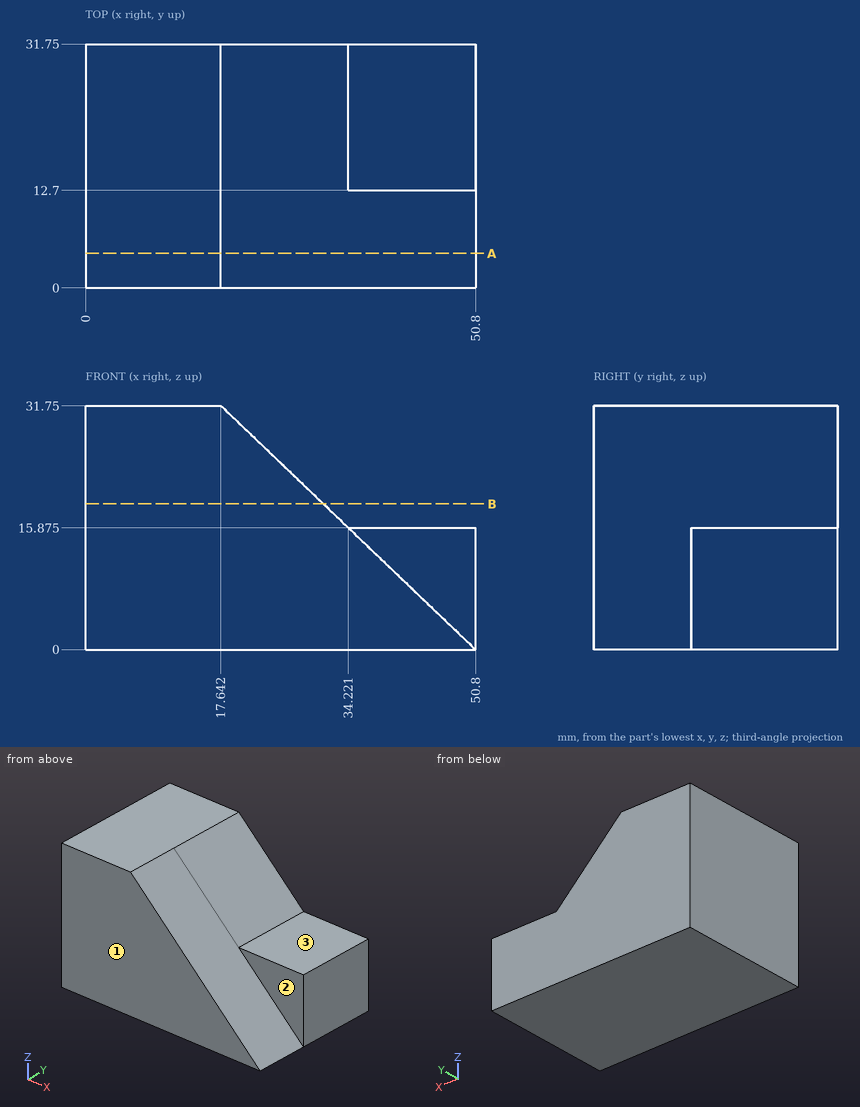
Design review of the part shown in the three views and the two pictorial views. Dimensions are in mm from the part's minimum x, y and z. A direction names the side the tool comes from. Round coordinates to 2 decimals unless told otherwise and drop trailing zeros. Loops run counter-clockwise (first coordinate to the right, second up) from the corner with the lowest first, then second, coordinate; pieces in that order, holes last. Notation, with made-up numbers: (68, 79.25) -> (116, 79.25) arc R19 cw to (116, 115.25) -> close; hole circle Ø3 at (-35, -32.5). An arc over 180 degrees is marked (long way). Answer as CSV lines item,"result".
1) Add section B-B on z = 19. Write out the cut boundary in (x, y), plus the area to 3 significant figures.
Geometry results:
outline,"(0, 0) -> (30.96, 0) -> (30.96, 31.75) -> (0, 31.75) -> close"
area,"983 mm²"
2) To check wall thickness, follow line 1 along Z through (x, y) = (36.5, 21) (1 decimal); line 2 along Z through (x, y) = (24.5, 10.5) (1 decimal); line 3 along X through (y, z) = (23, 29) (1 decimal). State the ranges of each line that lie inside material, in increasing order. Write a range as from..to.
Geometry results:
line 1,"z = 0..15.9"
line 2,"z = 0..25.2"
line 3,"x = 0..20.5"
3) Add section A-A on y = 4.5. Write out the cut boundary in (x, z).
Geometry results:
outline,"(0, 0) -> (50.8, 0) -> (17.64, 31.75) -> (0, 31.75) -> close"
4) For P1, Ø1, axis at y = 5.5, z = 15, coming from the +X side; P2, Ø2, axis at x = 21.5, y = 12.5, coming from the +Z side (1 decimal); P3, Ø13.5, axis at x = 46, y = 23.5, coming from the +Z side (3 decimals), all flat-tipped, find the tip position at first contact; note any pin that passes through.
Geometry results:
P1,"stops at x = 35.66"
P2,"stops at z = 29"
P3,"stops at z = 15.875"
5) Tool access review of the marked faces 1, 2 and 3: name each direction out of +Z, -Z, +X, -X, +Y, -Y from which nothing blocks a thin tool from reaching the whole face with its end or side.
Geometry results:
face 1,"+Z, -Z, +X, -X, -Y"
face 2,"+Z, +X, -Y"
face 3,"+Z, +X, +Y, -Y"
